from build123d import *

# Parameters (mm, degrees)
F1_DEPTH       = 20
F3_D           = 3.3
F3_CSINK_D     = 6.72
F3_CSINK_ANGLE = 90
F4_SIZE        = 2


with BuildPart() as f1:
    # F0 (on Front) → F1 (new body, symmetric)
    with BuildSketch(Plane.XZ):
        Polygon((-31, 4), (-31, 0), (-6, 0), (-6, -3.5), (0, -3.5), (0, 4), align=None)
    extrude(amount=F1_DEPTH, both=True)

    # F3 (through all)
    with Locations(Plane(origin=(0, 0, 0), x_dir=(1, 0, 0), z_dir=(0, 0, -1))):
        with Locations((-13, -13), (-24, 0), (-13, 13)):
            CounterSinkHole(F3_D / 2, F3_CSINK_D / 2, counter_sink_angle=F3_CSINK_ANGLE)

    # F4
    f4_edges = [f1.edges().sort_by_distance(p)[0] for p in [
        (-18.5, -20, 0),
        (-31, 0, 0),
        (-18.5, 20, 0),
        (-3, -20, -3.5),
        (-3, 20, -3.5),
        (0, 0, -3.5),
    ]]
    chamfer(f4_edges, length=F4_SIZE)


solid = f1.part
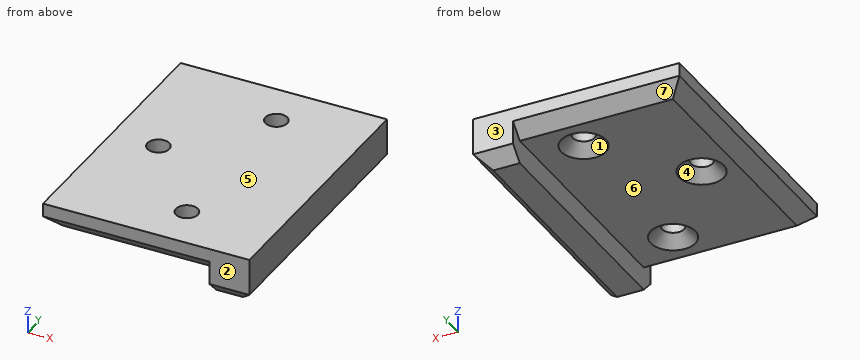
Geometry: final body of the model. Coordinates: model frame, mm. Face numbers are marked on the shaded views. A direction names the side the tool comes from. Give positions to 0.01 mm unless a question says otherwise; leave off trailing zeros. Write each loop counter-clockwise with the first axis right and the second up, starting at its lowest first coordinate (ties: lowest second). Pieces come first, ordered by that corner, then holes.
(1) Ray query, line 1 (Y direction, x = -13, z = 3.2); line 2 (Z direction, x = -19.5, y = -2); line 3 (X direction, y = 13, z = 2.3). Return the intervals inside material, ascending.
(2) First-contact query: P1, Ø4.5, axis at x = -13, y = -13, coming from the -Z side; P2, Ø4, axis at x = -12.5, y = 2, coming from the -Z side; P3, Ø3, axis at y = -0.5, z = -2, coming from the -X side; P4, Ø2.5, axis at x = -13, y = 13, coming from the +Z side. Flat tips, straight axial feed; report the tip coordinate or a pass-through.
(3) Cut plane A-A, the plane x = -24. Return loops of the section in (y, z).
(4) Cut plane C-C, the plane y = -9. Return loops of the section in (x, z), then the cut area to 3 significant figures.
(5) Mould query, pull axis Y, two halves, no side actions, for the marked faces 1, 2, 3 and 4. Classes: released by +Y, released by -Y, zero draft, split by the parting line, or undercut.
(6) Access query for the marked faces 5, 6 and 7. Directions: +Z, -Z, +X, -X, +Y, -Y. A direction counts if a zero-diameter tool reaches every point of the face in a straight line with its end or side. Return the directions, or none.
(7) Cut plane B-B, the plane y = -13. Return loops of the section in (x, z).
(8) Cut plane D-D, the plane z = -2. Return loops of the section in (x, y).
Values follow:
1. line 1: y = -20 to -14.65, -11.35 to 11.35, 14.65 to 20
1. line 2: z = 0 to 4
1. line 3: x = -31 to -14.65, -11.35 to 0
2. P1: stops at z = 1.11
2. P2: stops at z = 0
2. P3: stops at x = -6
2. P4: passes through
3. outline: (-20, 2) - (-18, 0) - (-3.36, 0) - (-1.65, 1.71) - (-1.65, 4) - (-20, 4) - close; (1.65, 1.71) - (3.36, 0) - (18, 0) - (20, 2) - (20, 4) - (1.65, 4) - close
4. outline: (-31, 2) - (-29, 0) - (-6, 0) - (-6, -3.5) - (-2, -3.5) - (0, -1.5) - (0, 4) - (-31, 4) - close
4. area: 141 mm2
5. face 1: undercut
5. face 2: released by -Y
5. face 3: released by +Y
5. face 4: undercut
6. face 5: +Z, +X, -X, +Y, -Y
6. face 6: -Z, -X, +Y, -Y
6. face 7: -Z, -X, +Y
7. outline: (-31, 2) - (-29, 0) - (-16.36, 0) - (-14.65, 1.71) - (-14.65, 4) - (-31, 4) - close; (-11.35, 1.71) - (-9.64, 0) - (-6, 0) - (-6, -3.5) - (-2, -3.5) - (0, -1.5) - (0, 4) - (-11.35, 4) - close
8. outline: (-6, -19.5) - (-0.5, -19.5) - (-0.5, 19.5) - (-6, 19.5) - close
